from build123d import *

# Parameters (mm, degrees)
SKETCH_1_R          = 4.4
EXTRUDE_1_DEPTH     = 0.7
SKETCH_2_R          = 3.35
EXTRUDE_2_DEPTH     = 1
SKETCH_3_R          = 3.4
EXTRUDE_3_DEPTH     = 1.9
SKETCH_4_R          = 10.526345736
SKETCH_4_R_2        = 3.3
CUT_EXTRUDE_1_DEPTH = 1
SKETCH_6_R          = 2
EXTRUDE_4_DEPTH     = 5


with BuildPart() as part:
    # 草图1 → 凸台-拉伸1 (new body)
    with BuildSketch(Plane(origin=(0, 0, 0), x_dir=(1, 0, 0), z_dir=(0, 1, 0))):
        Circle(SKETCH_1_R)
    extrude(amount=EXTRUDE_1_DEPTH)

    # 草图2 → 凸台-拉伸2 (add)
    with BuildSketch(Plane(origin=(0, 0.7, 0), x_dir=(1, 0, 0), z_dir=(0, 1, 0))):
        Circle(SKETCH_2_R)
    extrude(amount=EXTRUDE_2_DEPTH)

    # 草图3 → 凸台-拉伸3 (add)
    with BuildSketch(Plane(origin=(0, 1.7, 0), x_dir=(1, 0, 0), z_dir=(0, 1, 0))):
        Circle(SKETCH_3_R)
    extrude(amount=EXTRUDE_3_DEPTH)

    # 草图4 → 切除-拉伸1 (cut)
    with BuildSketch(Plane.XZ.offset(-1.7)):
        Circle(SKETCH_4_R)
        Circle(SKETCH_4_R_2, mode=Mode.SUBTRACT)
    extrude(amount=-CUT_EXTRUDE_1_DEPTH, mode=Mode.SUBTRACT)

    # 草图6 → 凸台-拉伸4 (add)
    with BuildSketch(Plane.XZ):
        Circle(SKETCH_6_R)
    extrude(amount=EXTRUDE_4_DEPTH)

    # 草图8 → 切除-旋转3 (revolve, cut)
    with BuildSketch(Plane(origin=(0, 0, 0), x_dir=(0, 0, -1), z_dir=(1, 0, 0))):
        with BuildLine():
            Line((0, 4.687391613), (0, 3.6))
            ThreePointArc((0, 3.6), (3.540607137, 2.39280141), (5.606264331, -0.72589827))
            Line((5.606264331, -0.72589827), (5.606264331, 4.687391613))
            Line((5.606264331, 4.687391613), (0, 4.687391613))
        make_face()
    revolve(axis=Axis((0, 3.6, 0), (0, -1, 0)), mode=Mode.SUBTRACT)


solid = part.part
For this review, take the finished solid that the model builds, in its own axes (mm). A direction names the side the tool comes from. Give positions to 0.01 mm unless a question says otherwise; leave off trailing zeros. Order: outer loops, then holes, each group sorted by start corner. A loop starts at its lowest first (then second) coordinate and runs counter-clockwise, first axis right, second up. Notation, with made-up numbers: M 69.25,54 L 110.25,54 A24 cw 110.25,84 Z; hole C -25,60.25 d9. An arc over 180 degrees is marked long. Answer in a Markdown table with one row per item. Add a question column.
(1) For pin 1 (2 mm diameter, centred on y = -1.5, z = -1.5, fed in from +X); pin 2 (2 mm diameter, centred on x = -3, z = -0.5, fed in from +Y); pin 3 (4 mm diameter, centred on x = 3, z = 3.5, fed in from +Y), all flat-tipped, find the tip position at first contact; note any pin that passes through.
(2) Consider section A-A on x = 0. State the section outline as (y, z) points.
(3) Consider section B-B on z = 0. State the section outline as (x, y) points.
(4) Consider section D-D on x = -1.5. State the section outline as (y, z) points.
(5) Consider section C-C on y = -1.5. State the section outline as (x, z) points, and give its area (3 significant figures).
(6) Wall thickness on probe 1 along Y at (x, z) = (-2.5, -3); probe 2 along Z at (x, y) = (0, -3.25); probe 3 along Z at (x, y) = (-1.5, 1.25): over which ranges is each line inside the solid? List them lowest first. Write a range as [from, to].
(7) For faces 1 (the face through (-2.43, 2.13, 2.23)), 2 (the face through (0, -2, -2)), 3 (the face through (4.197, 0.345, -1.322)), list the 3-axis set-ups (+Z, -Z, +X, -X, +Y, -Y) from which the entire face can be reached by the end or side of a thin tool; tool diameter is ignored.
Evaluation:
| question | item | result |
|---|---|---|
| 1 | pin 1 | stops at x = 1.94 |
| 1 | pin 2 | stops at y = 3.23 |
| 1 | pin 3 | stops at y = 2.98 |
| 2 | outline | M -5,-2 L 0,-2 L 0,-4.4 L 0.7,-4.4 L 0.7,-3.35 L 1.7,-3.35 L 1.7,-3.3 L 2.57,-3.3 A5.8 ccw 2.57,3.3 L 1.7,3.3 L 1.7,3.35 L 0.7,3.35 L 0.7,4.4 L 0,4.4 L 0,2 L -5,2 Z |
| 3 | outline | M -4.4,0 L -2,0 L -2,-5 L 2,-5 L 2,0 L 4.4,0 L 4.4,0.7 L 3.35,0.7 L 3.35,1.7 L 3.3,1.7 L 3.3,2.57 A5.8 ccw -3.3,2.57 L -3.3,1.7 L -3.35,1.7 L -3.35,0.7 L -4.4,0.7 Z |
| 4 | outline | M -5,-1.32 L 0,-1.32 L 0,-4.14 L 0.7,-4.14 L 0.7,-3 L 1.7,-3 L 1.7,-2.94 L 2.57,-2.94 A5.6 ccw 2.57,2.94 L 1.7,2.94 L 1.7,3 L 0.7,3 L 0.7,4.14 L 0,4.14 L 0,1.32 L -5,1.32 Z |
| 5 | outline | C 0,0 d4 |
| 5 | area | 12.6 mm^2 |
| 6 | probe 1 | y = [0, 0.7] |
| 6 | probe 2 | z = [-2, 2] |
| 6 | probe 3 | z = [-3, 3] |
| 7 | face 1 | +Y |
| 7 | face 2 | -Y |
| 7 | face 3 | +Y, -Y |
